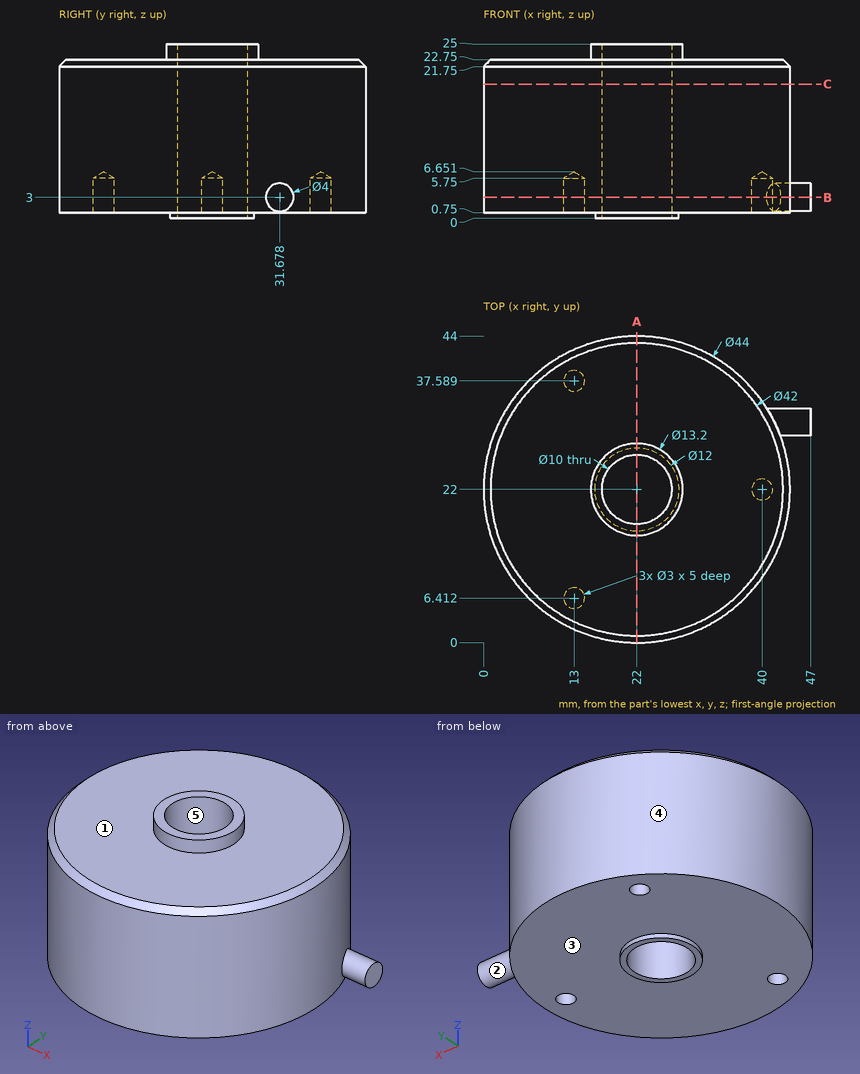
Source: three-view drawing plus pictorial views. Frame: mm from the lowest corner of the part. A direction names the side the tool comes from. Round coordinates to 2 decimals unless told otherwise and drop trailing zeros. Order: outer loops, then holes, each group sorted by start corner. A loop starts at its lowest first (then second) coordinate and runs counter-clockwise, first axis right, second up. Notation, with made-up numbers: (59, 67.25) -> (99, 67.25) arc R16 cw to (99, 71.25) -> close; hole circle Ø9 at (11.25, 22). An arc over 180 degrees is marked (long way). Use one line per item in the form item = value.
(1) Section C-C on z = 19.25. Return loops of the section in (x, y).
Results list:
outline = circle Ø44 at (22, 22); hole circle Ø10 at (22, 22)
(2) Section B-B on z = 3. Return loops of the section in (x, y) (1 decimal).
Results list:
outline = (40.6, 33.7) arc R22 ccw (long way) to (42.6, 29.7) -> (47, 29.7) -> (47, 33.7) -> close; hole circle Ø3 at (13, 6.4); hole circle Ø3 at (13, 37.6); hole circle Ø10 at (22, 22); hole circle Ø3 at (40, 22)
(3) First-contact query: pin 1 Ø3 at (y, z) = (27.5, 9.5) entering from -X; pin 2 Ø10 at (y, z) = (11.5, 3) entering from +X; pin 3 Ø1.5 at (x, y) = (18.5, 29) entering from +Z. Flat tips, straight axial feed; report the tip coordinate or a pass-through.
Results list:
pin_1 = 0.37
pin_2 = 43.3
pin_3 = 22.75
(4) Section A-A on x = 22. Return loops of the section in (y, z).
Results list:
outline = (0, 0.75) -> (16, 0.75) -> (16, 0) -> (17, 0) -> (17, 25) -> (15.4, 25) -> (15.4, 22.75) -> (1, 22.75) -> (0, 21.75) -> close; (27, 0) -> (28, 0) -> (28, 0.75) -> (44, 0.75) -> (44, 21.75) -> (43, 22.75) -> (28.6, 22.75) -> (28.6, 25) -> (27, 25) -> close
(5) Draft query along X for the marked faces 3, 4 and 5. Return one class per face: pulls with the +X half, pulls with the -X half, needs draft (parallel to the pull), parting line crosses it, or undercut.
Results list:
face_3 = needs draft
face_4 = parting line crosses it
face_5 = undercut
(6) Access query for the marked faces 1 and 2. Directions: +Z, -Z, +X, -X, +Y, -Y. A direction counts if a zero-diameter tool reaches every point of the face in a straight line with its end or side. Return the directions, or none.
Results list:
face_1 = +Z
face_2 = +X
(7) Ray query, probe 1 along Z at (x, y) = (18, 15); probe 2 along Y at (x, z) = (19, 18.5) (1 decimal); probe 3 along Y at (x, z) = (18.5, 22.5). Return the intervals inside material, ascending. Write a range as [from, to].
Results list:
probe_1 = [0.75, 22.75]
probe_2 = [0.2, 18], [26, 43.8]
probe_3 = [1.04, 18.43], [25.57, 42.96]
